Part model, mm, in its own coordinate system. A direction names the side the tool comes from. Coordinates: 2 decimals unless noted, no trailing zeros. Order: outer loops, then holes, each group sorted by start corner. A loop starts at its lowest first (then second) coordinate and runs counter-clockwise, first axis right, second up. Notation, with made-up numbers: (25.25, 23) - (36.25, 23) arc R24 cw to (36.25, 48) - close; hole circle Ø7 at (34.25, 67.5). An arc over 180 degrees is marked (long way). Use a Markdown table: item, result. Add a question column.
1) Saw through at C-C on y = -61. List the corners of the cut face in (x, z).
2) Two-plate mould, pull along Y, no slides. Class faces 1 (the face through (3.47, 4.47, -0.41)), 2 (the face through (0.031, 12.064, -0.082)), 3 (the face through (-1.905, -97, 0)): +Y half, -Y half, draft (parallel to the pull), parting line (faces both ways), or undercut.
3) Tool access for faces 4 (the face through (4.762, 9, 1)), 5 (the face through (-7.75, -86.48, -1.72)), 6 (the face through (3, -88.9, -1)): list every direction of +Z, -Z, +X, -X, +Y, -Y with a clear straight run to the whole face (end or side of a thin tool).
4) Wall check: L1, parallel to Y at x = 5, z = 0 (3 decimals); L2, parallel to Y at x = 0.75, z = 3.5; L3, parallel to Z at x = 2.75, y = 6.5. Give the ranges that are in metal, low to high. Write a range as [from, to].
5) Drop flat-ended pins along their axis: P1, Ø4, axis at y = -95.57, z = 0, coming from the +X side (3 decimals); P2, Ø2, axis at x = 0.5, z = -1.5, coming from the -Y side; P3, Ø5, axis at x = 2.5, y = -6.5, coming from the -Z side; P4, Ø4, axis at y = -52, z = 4.5, coming from the -X side. Give the stop position or say it passes through.
6) Saw through at B-B on y = 7.62. List the corners of the cut face in (x, z) (1 decimal).
7) Saw through at D-D on y = -13.5. List the corners of the cut face in (x, z).
8) Saw through at A-A on z = 0. Count the separate pieces of the cut face and the enclosed holes in it, then the cut area to 3 significant figures.
```python
from build123d import *

# Parameters (mm, degrees)
SKETCH1_R          = 7.9375
EXTRUDE1_DEPTH     = 86.995
SKETCH4_R          = 1.27
EXTRUDE2_DEPTH     = 2.2225
SKETCH5_R          = 5.3975
SKETCH5_R_2        = 1.27
EXTRUDE3_DEPTH     = 1.905
SKETCH6_R          = 4.1275
EXTRUDE4_DEPTH     = 1.905
SKETCH7_R          = 2.8575
EXTRUDE5_DEPTH     = 1.905
SKETCH8_R          = 3.175
SKETCH8_R_2        = 1.27
EXTRUDE6_DEPTH     = 2.54
SKETCH10_R         = 7.9375
SKETCH10_R_2       = 6.35
CUT_EXTRUDE2_DEPTH = 38.1
SKETCH11_R         = 7.9375
SKETCH11_R_2       = 1.27
CUT_EXTRUDE3_DEPTH = 48.26


with BuildPart() as part:
    # Sketch1 → Extrude1 (new body)
    with BuildSketch(Plane(origin=(0, 0, 0), x_dir=(1, 0, 0), z_dir=(0, 1, 0))):
        with Locations(Location((0, 0, 0), (0, 0, 270))):
            Circle(SKETCH1_R)
    extrude(amount=-EXTRUDE1_DEPTH)

    # Loft1: read off the stored shape, not the designer's step
    # Loft1: loft between two sections, ruled curve by curve
    loft1_from = [
        Edge.make_bspline([(3.207196431, 0, 7.26070226), (17.72860095, 0, 0.846309398), (11.314208088, 0, -13.675095122), (-3.207196431, 0, -7.26070226), (-17.72860095, 0, -0.846309398), (-11.314208088, 0, 13.675095122), (3.207196431, 0, 7.26070226)], [0, 0, 0, 0, 0.5, 0.5, 0.5, 1, 1, 1, 1], 3, [1, 0.333333333, 0.333333333, 1, 0.333333333, 0.333333333, 1]),
    ]
    loft1_to = [
        Edge.make_bspline([(0.075387957, 3.937, 1.903507724), (3.882403406, 3.937, 1.75273181), (3.731627491, 3.937, -2.054283639), (-0.075387957, 3.937, -1.903507724), (-3.882403406, 3.937, -1.75273181), (-3.731627491, 3.937, 2.054283639), (0.075387957, 3.937, 1.903507724)], [0, 0, 0, 0, 0.5, 0.5, 0.5, 1, 1, 1, 1], 3, [1, 0.333333333, 0.333333333, 1, 0.333333333, 0.333333333, 1]),
    ]
    loft1 = Solid(Shell([*[Face.make_surface_from_curves(loft1_from[k], loft1_to[k]) for k in range(1)], Face(Wire(loft1_from)), Face(Wire(loft1_to))]))
    add(loft1)

    # Sketch4 → Extrude2 (add, symmetric)
    with BuildSketch(Plane(origin=(0, 0, 0), x_dir=(0, 0, -1), z_dir=(1, 0, 0))):
        with BuildLine():
            Line((4.965601833, 1.905), (4.445, 8.89))
            ThreePointArc((4.445, 8.89), (0, 12.065), (-4.445, 8.89))
            Line((-4.445, 8.89), (-4.965601949, 1.905))
            Line((-4.965601949, 1.905), (-5.107584298, 0))
            Line((-5.107584298, 0), (5.107584151, 0))
            Line((5.107584151, 0), (4.965601833, 1.905))
        make_face()
        with Locations((0, 7.62)):
            Circle(SKETCH4_R, mode=Mode.SUBTRACT)
    extrude(amount=EXTRUDE2_DEPTH, both=True)

    # Sketch6 → Extrude4 (add)
    with BuildSketch(Plane.XZ.offset(86.995)):
        with Locations(Location((0, 0, 0), (0, 0, 90))):
            Circle(SKETCH6_R)
    extrude(amount=EXTRUDE4_DEPTH)



with BuildPart() as body_2:
    # Sketch5 → Extrude3 (new, symmetric)
    with BuildSketch(Plane(origin=(0, 0, 0), x_dir=(0, 0, -1), z_dir=(1, 0, 0))):
        with Locations(Location((0, -95.5675, 0), (0, 0, 180))):
            Circle(SKETCH5_R)
        with Locations(Location((0, -95.5675, 0), (0, 0, 180))):
            Circle(SKETCH5_R_2, mode=Mode.SUBTRACT)
    extrude(amount=EXTRUDE3_DEPTH, both=True)


with BuildPart() as part_1:
    add(part.part)

    add(body_2.part)  # Extrude5 merges body 2
    # Sketch7 → Extrude5 (add)
    with BuildSketch(Plane.XZ.offset(88.9)):
        with Locations(Location((0, 0, 0), (0, 0, 117.266044451))):
            Circle(SKETCH7_R)
    extrude(amount=EXTRUDE5_DEPTH)

    # Sketch8 → Extrude6 (add)
    with BuildSketch(Plane(origin=(2.2225, 0, 0), x_dir=(0, 0, -1), z_dir=(1, 0, 0))):
        with Locations(Location((0, 7.62, 0), (0, 0, 180))):
            Circle(SKETCH8_R)
        with Locations((0, 7.62)):
            Circle(SKETCH8_R_2, mode=Mode.SUBTRACT)
    extrude(amount=EXTRUDE6_DEPTH)

    # Sketch10 → Cut-Extrude2 (cut)
    with BuildSketch(Plane(origin=(0, -2.159, 0), x_dir=(-1, 0, 0), z_dir=(0, 1, 0))):
        with Locations(Location((0, 0, 0), (0, 0, 90))):
            Circle(SKETCH10_R)
        with Locations(Location((0, 0, 0), (0, 0, 90))):
            Circle(SKETCH10_R_2, mode=Mode.SUBTRACT)
    extrude(amount=-CUT_EXTRUDE2_DEPTH, mode=Mode.SUBTRACT)

    # Sketch11 → Cut-Extrude3 (cut)
    with BuildSketch(Plane(origin=(0, -37.719, 0), x_dir=(-1, 0, 0), z_dir=(0, 1, 0))):
        with Locations(Location((0, 0, 0), (0, 0, 90))):
            Circle(SKETCH11_R)
        with Locations(Location((0, 0, 0), (0, 0, 90))):
            Circle(SKETCH11_R_2, mode=Mode.SUBTRACT)
    extrude(amount=-CUT_EXTRUDE3_DEPTH, mode=Mode.SUBTRACT)


solid = part_1.part
```
Results are:
| question | item | result |
|---|---|---|
| 1 | outline | circle Ø2.54 at (0, 0) |
| 2 | face 1 | undercut |
| 2 | face 2 | +Y half |
| 2 | face 3 | draft |
| 3 | face 4 | +Z, -Z, +X, +Y |
| 3 | face 5 | +Y, -Y |
| 3 | face 6 | none |
| 4 | L1 | [-86.995, -85.979], [-37.719, 1.883] |
| 4 | L2 | [-99.68, -91.46], [-88.9, -85.98], [-37.72, 10.5] |
| 4 | L3 | [-2.97, -0.6], [0.6, 2.97] |
| 5 | P1 | x = 1.905 |
| 5 | P2 | y = -100.94 |
| 5 | P3 | z = -6.35 |
| 5 | P4 | through |
| 6 | outline | (-2.2, -4.5) - (2.2, -4.5) - (2.2, -3.2) - (4.8, -3.2) - (4.8, -1.3) - (-2.2, -1.3) - close; (-2.2, 1.3) - (4.8, 1.3) - (4.8, 3.2) - (2.2, 3.2) - (2.2, 4.5) - (-2.2, 4.5) - close |
| 7 | outline | circle Ø12.7 at (0, 0) |
| 8 | separate pieces | 3 |
| 8 | enclosed holes | 0 |
| 8 | area | 753 mm2 |
